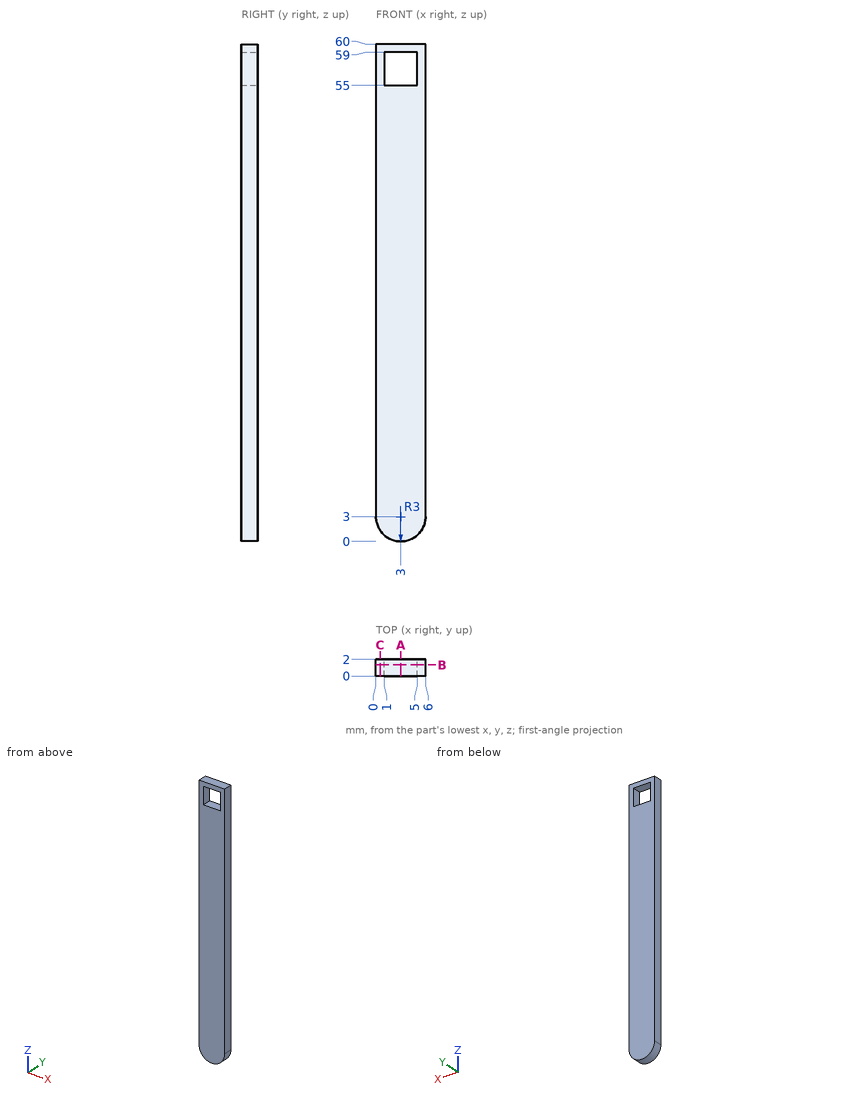
Could you check a few things on this drawing? It's one solid part, dimensions in mm from its lowest x, y, z. Coordinates: 2 decimals unless noted, no trailing zeros. Order: outer loops, then holes, each group sorted by start corner. A loop starts at its lowest first (then second) coordinate and runs counter-clockwise, first axis right, second up. Notation, with made-up numbers: M -36,-24 L 1,-24 A20 ccw 1,-1 Z; hole C 14.25,-4 d1. An arc over 180 degrees is marked long. Use a Markdown table: item, result. Add a question column.
Q1. I want a section at C-C on x = 0.5. List the corners of the cut face in (y, z) for me, then the cut area to 3 significant figures.
Q2. I want a section at A-A on x = 3. List the corners of the cut face in (y, z) for me.
Q3. If I drill on L1, parallel to Z at x = 3.2, y = 0.4; L2, parallel to Z at x = 4.9, y = 0.35; L3, parallel to Z at x = 5.35, y = 1.5, over which ranges is the centre line in solid material (lowest first)?
Q4. I want a section at B-B on y = 1.35. List the corners of the cut face in (x, z) for me, then the cut area to 3 significant figures.
Checked values:
| question | item | result |
|---|---|---|
| 1 | outline | M 0,1.34 L 2,1.34 L 2,60 L 0,60 Z |
| 1 | area | 117 mm² |
| 2 | outline | M 0,0 L 2,0 L 2,55 L 0,55 Z; M 0,59 L 2,59 L 2,60 L 0,60 Z |
| 3 | L1 | 0.01 to 55, 59 to 60 |
| 3 | L2 | 0.68 to 55, 59 to 60 |
| 3 | L3 | 1.14 to 60 |
| 4 | outline | M 0,3 A3 ccw 6,3 L 6,60 L 0,60 Z; hole M 1,55 L 5,55 L 5,59 L 1,59 Z |
| 4 | area | 340 mm² |
